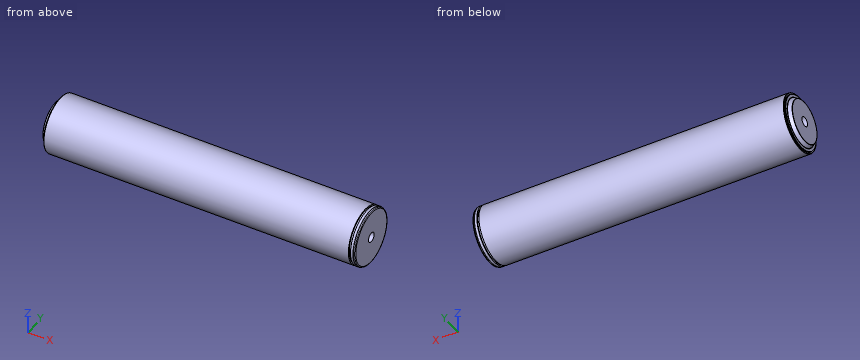
```python
from build123d import *


with BuildPart() as part:
    # Sketch1 → Base-Revolve (revolve)
    with BuildSketch(Plane.XY):
        with BuildLine():
            Line((163, 30), (0, 30))
            Line((0, 30), (-162.6, 30))
            ThreePointArc((-162.6, 30), (-162.882842712, 29.882842712), (-163, 29.6))
            Line((-163, 29.6), (-163, 28.4))
            ThreePointArc((-163, 28.4), (-163.117157288, 28.117157288), (-163.4, 28))
            Line((-163.4, 28), (-164, 28))
            Line((-164, 28), (-164, 25.230940108))
            ThreePointArc((-164, 25.230940108), (-164.053589838, 25.030940108), (-164.2, 24.884529946))
            Line((-164.2, 24.884529946), (-167.8, 22.806068977))
            ThreePointArc((-167.8, 22.806068977), (-167.946410162, 22.659658816), (-168, 22.459658816))
            Line((-168, 22.459658816), (-168, 5.1))
            Line((-168, 5.1), (-148, 5.1))
            Line((-148, 5.1), (-145.055513627, 0))
            Line((-145.055513627, 0), (147.055513627, 0))
            Line((147.055513627, 0), (150, 5.1))
            Line((150, 5.1), (170, 5.1))
            Line((170, 5.1), (170, 28.471851993))
            ThreePointArc((170, 28.471851993), (169.819152044, 29.04542843), (169.342020143, 29.411544614))
            Line((169.342020143, 29.411544614), (168.165693163, 29.839692621))
            ThreePointArc((168.165693163, 29.839692621), (167.997321197, 29.884807753), (167.823673019, 29.9))
            Line((167.823673019, 29.9), (165.15, 29.9))
            Line((165.15, 29.9), (165.15, 28.5))
            Line((165.15, 28.5), (163, 28.5))
            Line((163, 28.5), (163, 30))
        make_face()
    revolve(axis=Axis((-168, 0, 0), (1, 0, 0)))


solid = part.part
```
The listing builds one solid part. Answer for the finished solid, in the listing's coordinates (mm). Give positions to 0.01 mm unless a question says otherwise; leave off trailing zeros. Loops run counter-clockwise (first coordinate to the right, second up) from the corner with the lowest first, then second, coordinate; pieces in that order, holes last. Notation, with made-up numbers: (-4, 52) - (16, 52) arc R19 cw to (16, 69) - close; hole circle Ø10 at (46.5, 22). An arc over 180 degrees is marked (long way). Return JSON: item names as keys, results as strings. Group by question number.
1. Straight lines are drawn through the part: line 1 (Z direction, x = -151.75, y = 0); line 2 (Z direction, x = 163.25, y = 0); line 3 (X direction, y = -13.5, z = 25). For each, find the intervals that lie inside material, in ascending order. Write a range as [from, to].
2. Find section A-A (x = 130.5). Write down the section's boundary in (y, z), then the cut area to 3 significant figures.
3. Given pin 1 Ø5 at (x, z) = (31, 5) entering from +Y; pin 2 Ø1 at (x, y) = (-3, 0) entering from +Z; pin 3 Ø3 at (y, z) = (19, -23) entering from -X, each flat-ended and moving along its own axis, determine where each tip first touches the part or whether it passes through.
Verdict:
{
 "1": {"line 1": "z = [-30, -5.1], [5.1, 30]", "line 2": "z = [-28.5, -5.1], [5.1, 28.5]", "line 3": "x = [-163, 170]"},
 "2": {"outline": "circle Ø60 at (0, 0)", "area": "2,830 mm^2"},
 "3": {"pin 1": "stops at y = 29.9", "pin 2": "stops at z = 30", "pin 3": "stops at x = -163.01"}
}
